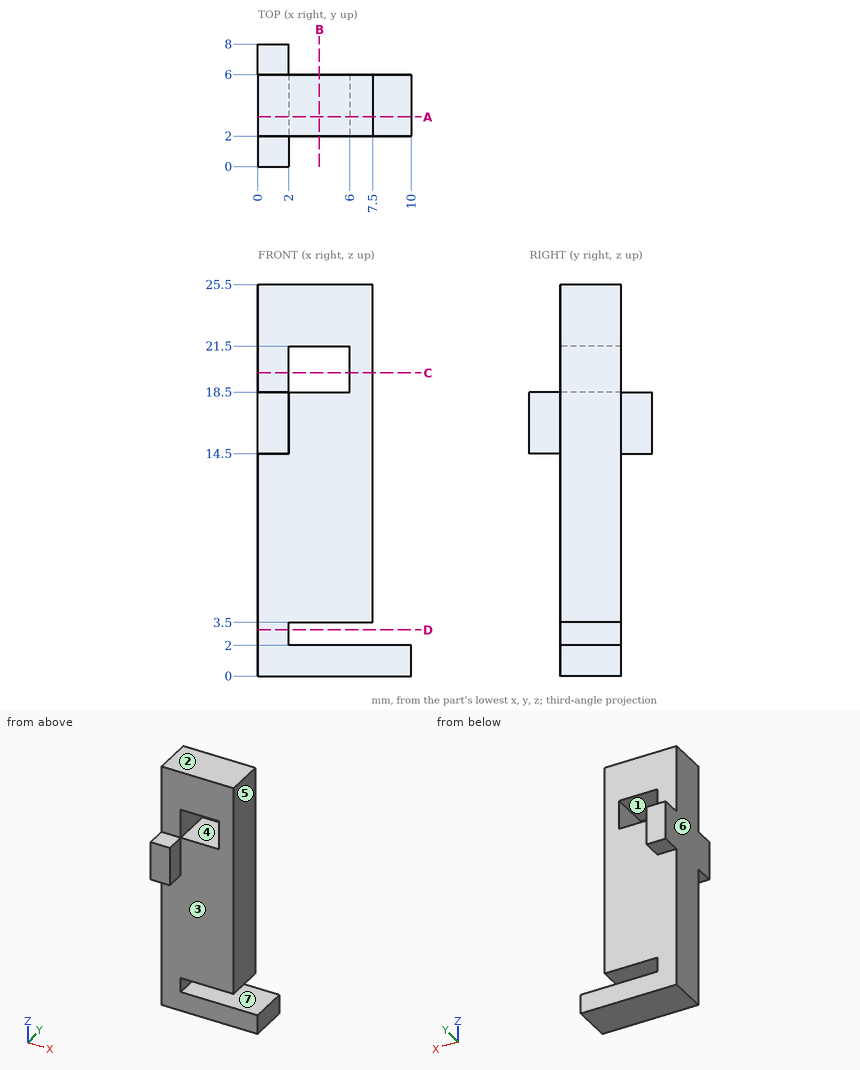
Can you work these out from the drawing? Everything is in mm from the part's minimum corner. A direction names the side the tool comes from. Round coordinates to 2 decimals unless told otherwise and drop trailing zeros. Write each loop counter-clockwise with the first axis right and the second up, starting at its lowest first coordinate (ties: lowest second). Pieces come first, ordered by that corner, then holes. Notation, with made-up numbers: M 59,59 L 97,59 A20 cw 97,91 Z; hole C 29,29 d6. An arc over 180 degrees is marked long. Use a Markdown table: item, result.
Item 1: I want a section at B-B (x = 4). List the corners of the cut face in (y, z) for me.
Found:
| item | result |
|---|---|
| outline | M 2,0 L 6,0 L 6,2 L 2,2 Z; M 2,3.5 L 6,3.5 L 6,18.5 L 2,18.5 Z; M 2,21.5 L 6,21.5 L 6,25.5 L 2,25.5 Z |
Item 2: If I drill on line 1 along Z through (x, y) = (5, 4.75); line 2 along X through (y, z) = (5.5, 20); line 3 along Y through (x, z) = (0.5, 22.5), over which ranges is the centre line in solid material (lowest first)? Write a range as [from, to].
Found:
| item | result |
|---|---|
| line 1 | z = [0, 2], [3.5, 18.5], [21.5, 25.5] |
| line 2 | x = [0, 2], [6, 7.5] |
| line 3 | y = [2, 6] |
Item 3: We'd pull the mould along Z, two halves only. Please class the marked faces 1, 2, 3 and 4: released by +Z, released by -Z, zero draft, split by the parting line, or undercut.
Found:
| item | result |
|---|---|
| face 1 | undercut |
| face 2 | released by +Z |
| face 3 | zero draft |
| face 4 | undercut |
Item 4: Which directions (+Z, -Z, +X, -X, +Y, -Y) give clear straight access to the entire face, cutting with the end or side of a thin tool? Please do the marked faces 5, 6 and 7.
Found:
| item | result |
|---|---|
| face 5 | +Z, +X, +Y, -Y |
| face 6 | +Z, -Z, -X, +Y, -Y |
| face 7 | +X, +Y, -Y |
Item 5: I want a section at D-D (z = 3). List the corners of the cut face in (x, y) for me, and give its area (3 significant figures).
Found:
| item | result |
|---|---|
| outline | M 0,2 L 2,2 L 2,6 L 0,6 Z |
| area | 8.00 mm2 |
Item 6: I want a section at C-C (z = 19.75). List the corners of the cut face in (x, y) for me, and give its area (3 significant figures).
Found:
| item | result |
|---|---|
| outline | M 0,2 L 2,2 L 2,6 L 0,6 Z; M 6,2 L 7.5,2 L 7.5,6 L 6,6 Z |
| area | 14.0 mm2 |
Item 7: For pin 1 Ø4 at (y, z) = (3.5, 13) entering from +X; pin 2 Ø2 at (x, y) = (4, 3.5) entering from -Z; pin 3 Ø5 at (x, z) = (5, 15.5) entering from -Y; pin 4 Ø3 at (x, z) = (3.5, 9.5) entering from +Y, each with a flat end and sliding along its axis, tell me the tip position at first contact or that it passes through.
Found:
| item | result |
|---|---|
| pin 1 | stops at x = 7.5 |
| pin 2 | stops at z = 0 |
| pin 3 | stops at y = 2 |
| pin 4 | stops at y = 6 |
Item 8: I want a section at A-A (y = 3.25). List the corners of the cut face in (x, z) for me, and give its area (3 significant figures).
Found:
| item | result |
|---|---|
| outline | M 0,0 L 10,0 L 10,2 L 2,2 L 2,3.5 L 7.5,3.5 L 7.5,25.5 L 0,25.5 Z; hole M 2,18.5 L 6,18.5 L 6,21.5 L 2,21.5 Z |
| area | 176 mm2 |
